Source: CAD feature listing. Evaluate the final solid. Frame: model axes, mm. Face numbers are marked on the shaded views. A direction names the side the tool comes from. Coordinates: 2 decimals unless noted, no trailing zeros. Loops run counter-clockwise (first coordinate to the right, second up) from the corner with the lowest first, then second, coordinate; pieces in that order, holes last.
from build123d import *

# Parameters (mm, degrees)
SKETCH1_W           = 157
SKETCH1_H           = 75
BOSS_EXTRUDE1_DEPTH = 38
SHELL1_T            = -2
FILLET1_R           = 3


with BuildPart() as part:
    # Sketch1 → Boss-Extrude1 (new body)
    with BuildSketch(Plane(origin=(0, 0, 0), x_dir=(1, 0, 0), z_dir=(0, 1, 0))):
        with Locations((-78.5, 37.5)):
            Rectangle(SKETCH1_W, SKETCH1_H)
    extrude(amount=BOSS_EXTRUDE1_DEPTH)

    # Shell1
    shell1_openings = [part.faces().sort_by_distance(p)[0] for p in [
        (-78.5, 38, -37.5),
    ]]
    offset(amount=SHELL1_T, openings=shell1_openings, kind=Kind.INTERSECTION)

    # Fillet1
    fillet1_edges = [part.edges().sort_by_distance(p)[0] for p in [
        (-2, 20, -2),
        (-2, 20, -73),
        (-155, 20, -73),
        (-155, 20, -2),
        (0, 19, 0),
        (-157, 19, 0),
        (-157, 19, -75),
        (0, 19, -75),
    ]]
    fillet(fillet1_edges, radius=FILLET1_R)


solid = part.part
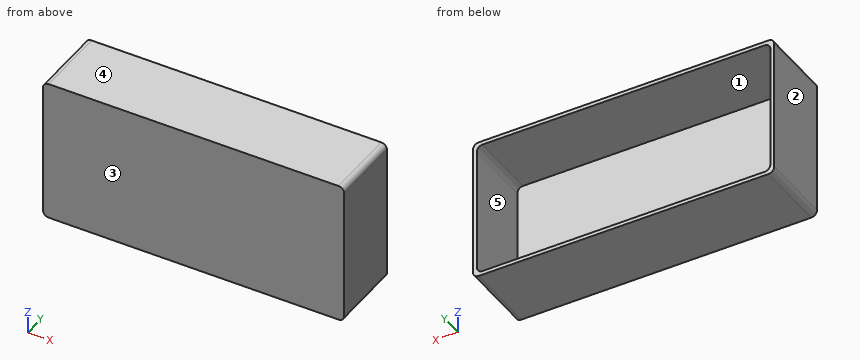
Q1. Access query for the marked faces 1 and 2. Directions: +Z, -Z, +X, -X, +Y, -Y. A direction counts if a zero-diameter tool reaches every point of the face in a straight line with its end or side. Return the directions, or none.
Q2. Line query: line 1 along X through (y, z) = (24.5, -10.5); line 2 along Z through (x, y) = (-6.5, 7); line 3 along Y through (x, z) = (-60, -53). Output: solid intervals per line, ascending.
Q3. Section A-A, the plane y = 34.5. Return the cut outline in (x, z), plus the area to 3 significant figures.
Q4. Section B-B, the plane z = -67. Return the cut outline in (x, y), plus the area to 3 significant figures.
Q5. Section C-C, the plane x = -134. Return the cut outline in (y, z).
Q6. Contact query for a flat-ended pin moving along its axis: pin 1 Ø21.5 at (x, z) = (-69.5, -35) entering from +Y. Output: stop coordinate, or through.
Q7. Draft query along Z for the marked faces 3, 4 and 5. Return one class per face: +Z half, -Z half, draft (parallel to the pull), parting line (faces both ways), or undercut.
Derived:
1. face 1: +Y
1. face 2: +Z, -Z, -X, +Y, -Y
2. line 1: x = -157 to -155, -2 to 0
2. line 2: z = -75 to -73, -2 to 0
2. line 3: y = 0 to 2
3. outline: (-157, -72) arc R3 ccw to (-154, -75) - (-3, -75) arc R3 ccw to (0, -72) - (0, -3) arc R3 ccw to (-3, 0) - (-154, 0) arc R3 ccw to (-157, -3) - close; hole (-155, -70) arc R3 ccw to (-152, -73) - (-5, -73) arc R3 ccw to (-2, -70) - (-2, -5) arc R3 ccw to (-5, -2) - (-152, -2) arc R3 ccw to (-155, -5) - close
3. area: 912 mm2
4. outline: (-157, 0) - (0, 0) - (0, 38) - (-2, 38) - (-2, 2) - (-155, 2) - (-155, 38) - (-157, 38) - close
4. area: 458 mm2
5. outline: (0, -75) - (38, -75) - (38, -73) - (2, -73) - (2, -2) - (38, -2) - (38, 0) - (0, 0) - close
6. pin 1: stops at y = 2
7. face 3: draft
7. face 4: +Z half
7. face 5: undercut
